Check sheet for the modelled part. Datum: model origin and axes. Units: mm. A direction names the side the tool comes from. Round coordinates to 2 decimals unless told otherwise and drop trailing zeros. Loops run counter-clockwise (first coordinate to the right, second up) from the corner with the lowest first, then second, coordinate; pieces in that order, holes last. Notation, with made-up numbers: (58, 32) - (82, 32) arc R29 ccw to (82, 55) - close; hole circle Ø5 at (62, 8). An arc over 180 degrees is marked (long way). Put each result on its own line as item: value. Start each with the question number.
Item 1: Tool access check on faces 4 (the flat face through (36.408, -0.356, -11.344)), 5 (the flat face through (-20, 25.4, 24)), 6 (the flat face through (-85.499, -0.356, 17.133)), 7 (the flat face through (-44.25, -0.36, 74.68)), 8 (the flat face through (36.29, -0.36, 1.24)). Record the directions out of +Z, -Z, +X, -X, +Y, -Y that give a thin tool (end or side, any length) a straight path to the whole face; none if there is none.
Item 2: Section check D-D, the plane z = 15.5. Record the cut outline in (x, y).
Item 3: Section check C-C, the plane y = 8.5. Record the cut outline in (x, z), and give its area (3 significant figures).
Item 4: Gauge pin test, flat ends, axial feed: pin 1 Ø8 at (x, y) = (-91.5, -6.5) entering from +Z; pin 2 Ø10 at (x, y) = (44.5, -12.5) entering from +Z; pin 3 Ø8 at (x, y) = (-68, -6.5) entering from -Z. Record the tip position at first contact, or that the pin passes through.
Item 5: Material ranges on line 1 along Z through (x, y) = (8.5, 21); line 2 along Z through (x, y) = (7.5, -10); line 3 along X through (y, z) = (-3.5, 93), recorded low to high.
Item 6: Section check A-A, the plane z = 69.5. Record the cut outline in (x, y).
Item 7: Draft check along X on faces 1 (the flat face through (-20, -25.4, 24)), 2 (the flat face through (15.47, -0.36, 66.08)), 3 (the flat face through (-59.48, -0.36, 65.55)). Enter one of: pulls with the +X half, pulls with the -X half, needs draft (parallel to the pull), parting line crosses it, or undercut.
Item 8: Section check B-B, the plane x = 48. Record the cut outline in (y, z), and give its area (3 significant figures).
from build123d import *

# Parameters (mm, degrees)
F1_DEPTH = 25.4


with BuildPart() as f1:
    # F0 (on Front) → F1 (new body, symmetric)
    with BuildSketch(Plane.XZ):
        Polygon((0, -7.260618), (2.209697, -0.688518), (71.577795, -22.302875), (0, 25.454371), (61.308518, 85.952409), (-31.664561, 45.646154), (-57.191979, 104.529388), (-61.833249, 25.454371), (-109.835885, 8.574612), (-38.279932, 0), (-16.56682, -56.533791), align=None)
    extrude(amount=F1_DEPTH, both=True)


solid = f1.part
Check result:
1. face 4: -Z, +Y, -Y
1. face 5: +Z, -Z, +X, -X, +Y
1. face 6: +Z, -X, +Y, -Y
1. face 7: +Z, +Y, -Y
1. face 8: +X, +Y, -Y
2. outline: (-90.14, -25.4) - (14.92, -25.4) - (14.92, 25.4) - (-90.14, 25.4) - close
3. outline: (-109.84, 8.57) - (-38.28, 0) - (-16.57, -56.53) - (2.21, -0.69) - (71.58, -22.3) - (0, 25.45) - (61.31, 85.95) - (-31.66, 45.65) - (-57.19, 104.53) - (-61.83, 25.45) - close
3. area: 7,490 mm²
4. pin 1: z = 16.43
4. pin 2: z = 80.83
4. pin 3: z = 3.08
5. line 1: -2.65 to 19.78, 33.84 to 63.06
5. line 2: -2.34 to 20.45, 32.86 to 62.63
5. line 3: -57.87 to -52.19
6. outline: (-59.25, -25.4) - (-42.01, -25.4) - (-42.01, 25.4) - (-59.25, 25.4) - close; (23.36, -25.4) - (44.64, -25.4) - (44.64, 25.4) - (23.36, 25.4) - close
7. face 1: needs draft
7. face 2: undercut
7. face 3: pulls with the -X half
8. outline: (-25.4, -14.96) - (25.4, -14.96) - (25.4, -6.57) - (-25.4, -6.57) - close; (-25.4, 72.82) - (25.4, 72.82) - (25.4, 80.18) - (-25.4, 80.18) - close
8. area: 800 mm²
